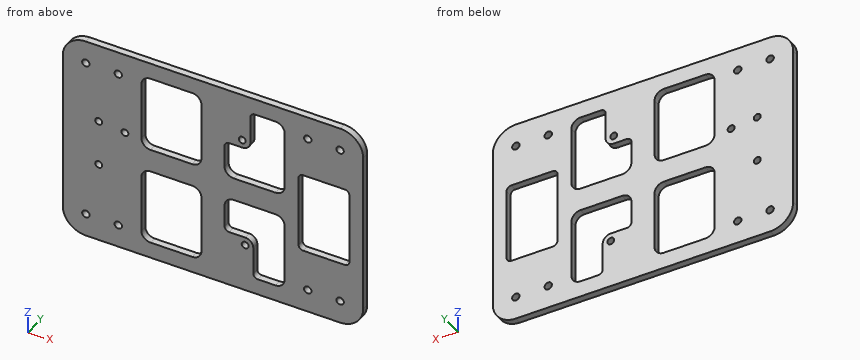
```python
from build123d import *

# Parameters (mm, degrees)
SKETCH2_W           = 130
SKETCH2_H           = 90
BOSS_EXTRUDE1_DEPTH = 3
SKETCH3_R           = 1.5
CUT_EXTRUDE1_DEPTH  = 10
SKETCH4_R           = 1.6
CUT_EXTRUDE2_DEPTH  = 10
FILLET1_R           = 10
CUT_EXTRUDE3_DEPTH  = 10
SKETCH6_R           = 1.5
BOSS_EXTRUDE4_DEPTH = 3
SKETCH6_6_R         = 1.5
CUT_EXTRUDE4_DEPTH  = 3
SKETCH8_R           = 1.5
CUT_EXTRUDE5_DEPTH  = 10
SKETCH9_W           = 22
SKETCH9_H           = 35
CUT_EXTRUDE6_DEPTH  = 10
FILLET2_R           = 2


with BuildPart() as part:
    # Sketch2 → Boss-Extrude1 (new body)
    with BuildSketch(Plane(origin=(0, 0, 0), x_dir=(1, 0, 0), z_dir=(0, 1, 0))):
        with Locations((71.271186441, 55.564971751)):
            Rectangle(SKETCH2_W, SKETCH2_H)
    extrude(amount=-BOSS_EXTRUDE1_DEPTH)

    # Sketch3 → Cut-Extrude1 (cut)
    with BuildSketch(Plane(origin=(0, 0, 0), x_dir=(1, 0, 0), z_dir=(0, 1, 0))):
        with Locations(Location((126.271186441, 63.564971751, 0), (0, 0, 270))):
            Circle(SKETCH3_R)
        with Locations(Location((126.271186441, 47.564971751, 0), (0, 0, 270))):
            Circle(SKETCH3_R)
        with Locations(Location((112.271186441, 47.564971751, 0), (0, 0, 270))):
            Circle(SKETCH3_R)
        with Locations(Location((112.271186441, 63.564971751, 0), (0, 0, 270))):
            Circle(SKETCH3_R)
        with Locations(Location((16.271186441, 47.564971751, 0), (0, 0, 90))):
            Circle(SKETCH3_R)
        with Locations(Location((30.271186441, 47.564971751, 0), (0, 0, 90))):
            Circle(SKETCH3_R)
        with Locations(Location((16.271186441, 63.564971751, 0), (0, 0, 90))):
            Circle(SKETCH3_R)
        with Locations(Location((30.271186441, 63.564971751, 0), (0, 0, 90))):
            Circle(SKETCH3_R)
    extrude(amount=-CUT_EXTRUDE1_DEPTH, mode=Mode.SUBTRACT)

    # Sketch4 → Cut-Extrude2 (cut)
    with BuildSketch(Plane(origin=(0, 0, 0), x_dir=(1, 0, 0), z_dir=(0, 1, 0))):
        with Locations(Location((16.271186441, 20.564971751, 0), (0, 0, 270))):
            Circle(SKETCH4_R)
        with Locations(Location((30.271186441, 20.564971751, 0), (0, 0, 270))):
            Circle(SKETCH4_R)
        with Locations(Location((30.271186441, 90.564971751, 0), (0, 0, 90))):
            Circle(SKETCH4_R)
        with Locations(Location((16.271186441, 90.564971751, 0), (0, 0, 90))):
            Circle(SKETCH4_R)
        with Locations(Location((112.271186441, 20.564971751, 0), (0, 0, 90))):
            Circle(SKETCH4_R)
        with Locations(Location((126.271186441, 20.564971751, 0), (0, 0, 90))):
            Circle(SKETCH4_R)
        with Locations(Location((126.271186441, 90.564971751, 0), (0, 0, 270))):
            Circle(SKETCH4_R)
        with Locations(Location((112.271186441, 90.564971751, 0), (0, 0, 270))):
            Circle(SKETCH4_R)
    extrude(amount=-CUT_EXTRUDE2_DEPTH, mode=Mode.SUBTRACT)

    # Fillet1
    fillet1_edges = [part.edges().sort_by_distance(p)[0] for p in [
        (6.271186441, -1.5, -100.564971751),
        (136.271186441, -1.5, -100.564971751),
        (136.271186441, -1.5, -10.564971751),
        (6.271186441, -1.5, -10.564971751),
    ]]
    fillet(fillet1_edges, radius=FILLET1_R)

    # Sketch5 → Cut-Extrude3 (cut)
    with BuildSketch(Plane(origin=(0, 0, 0), x_dir=(1, 0, 0), z_dir=(0, 1, 0))):
        with BuildLine():
            Line((76.271186441, 89.564971751), (76.271186441, 64.564971751))
            ThreePointArc((76.271186441, 64.564971751), (77.442759316, 61.736544627), (80.271186441, 60.564971751))
            Line((80.271186441, 60.564971751), (98.271186441, 60.564971751))
            ThreePointArc((98.271186441, 60.564971751), (101.099613565, 61.736544627), (102.271186441, 64.564971751))
            Line((102.271186441, 64.564971751), (102.271186441, 89.564971751))
            ThreePointArc((102.271186441, 89.564971751), (101.099613565, 92.393398876), (98.271186441, 93.564971751))
            Line((98.271186441, 93.564971751), (80.271186441, 93.564971751))
            ThreePointArc((80.271186441, 93.564971751), (77.442759316, 92.393398876), (76.271186441, 89.564971751))
        make_face()
        with BuildLine():
            Line((40.271186441, 89.564971751), (40.271186441, 64.564971751))
            ThreePointArc((40.271186441, 64.564971751), (41.442759316, 61.736544627), (44.271186441, 60.564971751))
            Line((44.271186441, 60.564971751), (62.271186441, 60.564971751))
            ThreePointArc((62.271186441, 60.564971751), (65.099613565, 61.736544627), (66.271186441, 64.564971751))
            Line((66.271186441, 64.564971751), (66.271186441, 89.564971751))
            ThreePointArc((66.271186441, 89.564971751), (65.099613565, 92.393398876), (62.271186441, 93.564971751))
            Line((62.271186441, 93.564971751), (44.271186441, 93.564971751))
            ThreePointArc((44.271186441, 93.564971751), (41.442759316, 92.393398876), (40.271186441, 89.564971751))
        make_face()
        with BuildLine():
            Line((66.271186441, 21.564971751), (66.271186441, 46.564971751))
            ThreePointArc((66.271186441, 46.564971751), (65.099613565, 49.393398876), (62.271186441, 50.564971751))
            Line((62.271186441, 50.564971751), (44.271186441, 50.564971751))
            ThreePointArc((44.271186441, 50.564971751), (41.442759316, 49.393398876), (40.271186441, 46.564971751))
            Line((40.271186441, 46.564971751), (40.271186441, 21.564971751))
            ThreePointArc((40.271186441, 21.564971751), (41.442759316, 18.736544627), (44.271186441, 17.564971751))
            Line((44.271186441, 17.564971751), (62.271186441, 17.564971751))
            ThreePointArc((62.271186441, 17.564971751), (65.099613565, 18.736544627), (66.271186441, 21.564971751))
        make_face()
        with BuildLine():
            Line((102.271186441, 21.564971751), (102.271186441, 46.564971751))
            ThreePointArc((102.271186441, 46.564971751), (101.099613565, 49.393398876), (98.271186441, 50.564971751))
            Line((98.271186441, 50.564971751), (80.271186441, 50.564971751))
            ThreePointArc((80.271186441, 50.564971751), (77.442759316, 49.393398876), (76.271186441, 46.564971751))
            Line((76.271186441, 46.564971751), (76.271186441, 21.564971751))
            ThreePointArc((76.271186441, 21.564971751), (77.442759316, 18.736544627), (80.271186441, 17.564971751))
            Line((80.271186441, 17.564971751), (98.271186441, 17.564971751))
            ThreePointArc((98.271186441, 17.564971751), (101.099613565, 18.736544627), (102.271186441, 21.564971751))
        make_face()
    extrude(amount=-CUT_EXTRUDE3_DEPTH, mode=Mode.SUBTRACT)

    # Sketch6 → Boss-Extrude4 (add)
    # profile 1 of 10: a face of its own
    with BuildSketch(Plane(origin=(0, 0, 0), x_dir=(1, 0, 0), z_dir=(0, 1, 0))):
        with BuildLine():
            Line((87.436129721, 17.564971751), (87.436129721, 31.434971751))
            ThreePointArc((87.436129721, 31.434971751), (86.411003455, 33.909845486), (83.936129721, 34.934971751))
            Line((83.936129721, 34.934971751), (76.271186441, 34.934971751))
            Line((76.271186441, 34.934971751), (76.271186441, 17.564971751))
            Line((76.271186441, 17.564971751), (87.436129721, 17.564971751))
        make_face()
        with Locations(Location((83.936129721, 31.434971751, 0), (0, 0, 270))):
            Circle(SKETCH6_R, mode=Mode.SUBTRACT)
    # profile 2 of 10: a face of its own
    with BuildSketch(Plane(origin=(0, 0, 0), x_dir=(1, 0, 0), z_dir=(0, 1, 0))):
        with BuildLine():
            Line((88.706129721, 79.694971751), (88.706129721, 93.564971751))
            Line((88.706129721, 93.564971751), (76.271186441, 93.564971751))
            Line((76.271186441, 93.564971751), (76.271186441, 76.194971751))
            Line((76.271186441, 76.194971751), (85.206129721, 76.194971751))
            ThreePointArc((85.206129721, 76.194971751), (87.681003455, 77.220098017), (88.706129721, 79.694971751))
        make_face()
        with Locations(Location((85.206129721, 79.694971751, 0), (0, 0, 270))):
            Circle(SKETCH6_R, mode=Mode.SUBTRACT)
    # profile 3 of 10: a face of its own
    with BuildSketch(Plane(origin=(0, 0, 0), x_dir=(1, 0, 0), z_dir=(0, 1, 0))):
        with Locations((30.271186441, 47.564971751)):
            Circle(SKETCH6_R)
    # profile 4 of 10: a face of its own
    with BuildSketch(Plane(origin=(0, 0, 0), x_dir=(1, 0, 0), z_dir=(0, 1, 0))):
        with Locations((16.271186441, 47.564971751)):
            Circle(SKETCH6_R)
    # profile 5 of 10: a face of its own
    with BuildSketch(Plane(origin=(0, 0, 0), x_dir=(1, 0, 0), z_dir=(0, 1, 0))):
        with Locations((16.271186441, 63.564971751)):
            Circle(SKETCH6_R)
    # profile 6 of 10: a face of its own
    with BuildSketch(Plane(origin=(0, 0, 0), x_dir=(1, 0, 0), z_dir=(0, 1, 0))):
        with Locations((30.271186441, 63.564971751)):
            Circle(SKETCH6_R)
    # profile 7 of 10: a face of its own
    with BuildSketch(Plane(origin=(0, 0, 0), x_dir=(1, 0, 0), z_dir=(0, 1, 0))):
        with Locations((112.271186441, 47.564971751)):
            Circle(SKETCH6_R)
    # profile 8 of 10: a face of its own
    with BuildSketch(Plane(origin=(0, 0, 0), x_dir=(1, 0, 0), z_dir=(0, 1, 0))):
        with Locations((112.271186441, 63.564971751)):
            Circle(SKETCH6_R)
    # profile 9 of 10: a face of its own
    with BuildSketch(Plane(origin=(0, 0, 0), x_dir=(1, 0, 0), z_dir=(0, 1, 0))):
        with Locations((126.271186441, 63.564971751)):
            Circle(SKETCH6_R)
    # profile 10 of 10: a face of its own
    with BuildSketch(Plane(origin=(0, 0, 0), x_dir=(1, 0, 0), z_dir=(0, 1, 0))):
        with Locations((126.271186441, 47.564971751)):
            Circle(SKETCH6_R)
    extrude(amount=-BOSS_EXTRUDE4_DEPTH)

    # Sketch6<6> → Cut-Extrude4 (cut)
    with BuildSketch(Plane(origin=(0, 0, 0), x_dir=(1, 0, 0), z_dir=(0, 1, 0))):
        with Locations(Location((33.136129721, 46.674971751, 0), (0, 0, 270))):
            Circle(SKETCH6_6_R)
    extrude(amount=-CUT_EXTRUDE4_DEPTH, mode=Mode.SUBTRACT)

    # Sketch8 → Cut-Extrude5 (cut)
    with BuildSketch(Plane(origin=(0, 0, 0), x_dir=(1, 0, 0), z_dir=(0, 1, 0))):
        with Locations(Location((21.821186441, 65.564971751, 0), (0, 0, 270))):
            Circle(SKETCH8_R)
        with Locations(Location((21.821186441, 45.564971751, 0), (0, 0, 270))):
            Circle(SKETCH8_R)
    extrude(amount=-CUT_EXTRUDE5_DEPTH, mode=Mode.SUBTRACT)

    # Sketch9 → Cut-Extrude6 (cut)
    with BuildSketch(Plane(origin=(0, 0, 0), x_dir=(1, 0, 0), z_dir=(0, 1, 0))):
        with Locations((119.271186441, 55.564971751)):
            Rectangle(SKETCH9_W, SKETCH9_H)
    extrude(amount=-CUT_EXTRUDE6_DEPTH, mode=Mode.SUBTRACT)

    # Fillet2
    fillet2_edges = [part.edges().sort_by_distance(p)[0] for p in [
        (76.271186441, -1.5, -76.194971751),
        (88.706129721, -1.5, -93.564971751),
        (87.436129721, -1.5, -17.564971751),
        (76.271186441, -1.5, -34.934971751),
        (108.271186441, -1.5, -38.064971751),
        (108.271186441, -1.5, -73.064971751),
        (130.271186441, -1.5, -73.064971751),
        (130.271186441, -1.5, -38.064971751),
    ]]
    fillet(fillet2_edges, radius=FILLET2_R)


solid = part.part
```
Geometry check sheet. Reference: the model listing, model coordinates, mm. Coordinates: 2 decimals unless noted, no trailing zeros. Order: outer loops, then holes, each group sorted by start corner. A loop starts at its lowest first (then second) coordinate and runs counter-clockwise, first axis right, second up. Notation, with made-up numbers: M 80.25,11 L 130.25,11 A7 cw 130.25,20 Z; hole C 57.25,67 d10. An arc over 180 degrees is marked long. Answer as a JSON object with one key per item and string values.
Q1. Scan lines: line 1 (Z direction, x = 58, y = -0.85); line 2 (X direction, y = -2.55, z = -88.5); line 3 (X direction, y = -0.15, z = -26.5). Record each from-to range of solid material in increasing order.
Results are:
{"line 1": "z = -100.56 to -93.56, -60.56 to -50.56, -17.56 to -10.56", "line 2": "x = 6.27 to 40.27, 66.27 to 88.71, 102.27 to 136.27", "line 3": "x = 6.27 to 40.27, 66.27 to 87.44, 102.27 to 136.27"}
Q2. Cross-section at B-B on z = -84.5. Record the cut outline in (x, y), and give its area (3 significant figures).
Results are:
{"outline": "M 6.27,-3 L 40.27,-3 L 40.27,0 L 6.27,0 Z; M 66.27,-3 L 88.71,-3 L 88.71,0 L 66.27,0 Z; M 102.27,-3 L 136.27,-3 L 136.27,0 L 102.27,0 Z", "area": "271 mm²"}
Q3. Cross-section at A-A on x = 116.5. Record the cut outline in (y, z), and give its area (3 significant figures).
Results are:
{"outline": "M -3,-100.56 L 0,-100.56 L 0,-73.06 L -3,-73.06 Z; M -3,-38.06 L 0,-38.06 L 0,-10.56 L -3,-10.56 Z", "area": "165 mm²"}
Q4. Cross-section at D-D on z = -42. Record the cut outline in (x, y), and give its area (3 significant figures).
Results are:
{"outline": "M 6.27,-3 L 40.27,-3 L 40.27,0 L 6.27,0 Z; M 66.27,-3 L 76.27,-3 L 76.27,0 L 66.27,0 Z; M 102.27,-3 L 108.27,-3 L 108.27,0 L 102.27,0 Z; M 130.27,-3 L 136.27,-3 L 136.27,0 L 130.27,0 Z", "area": "168 mm²"}
Q5. Cross-section at C-C on x = 64. Record the cut outline in (y, z), and give its area (3 significant figures).
Results are:
{"outline": "M -3,-100.56 L 0,-100.56 L 0,-93.17 L -3,-93.17 Z; M -3,-60.96 L 0,-60.96 L 0,-50.17 L -3,-50.17 Z; M -3,-17.96 L 0,-17.96 L 0,-10.56 L -3,-10.56 Z", "area": "76.7 mm²"}
